CAD build for the part. Positions are in the model's coordinates, mm. Give positions to 0.01 mm unless a question says otherwise; leave off trailing zeros. Write each loop counter-clockwise with the first axis right and the second up, starting at its lowest first coordinate (ties: lowest second). Pieces come first, ordered by that corner, then holes. Notation, with made-up numbers: (-34, 6) - (-23, 6) arc R29 ccw to (-23, 36) - close; hole circle Ø4 at (-18.75, -39). An arc over 180 degrees is marked (long way). Answer as a JSON object with one key per item and string values.
from build123d import *

# Parameters (mm, degrees)
CROQUIS1_R              = 3
SALIENTE_EXTRUIR1_DEPTH = 5
REDONDEO1_R             = 2.99


with BuildPart() as part:
    # Croquis1 → Saliente-Extruir1 (new body)
    with BuildSketch(Plane(origin=(0, 0, 0), x_dir=(1, 0, 0), z_dir=(0, 1, 0))):
        with BuildLine():
            Line((-7.962657019, 208.875039065), (-0.868497325, 213.470388318))
            Line((-0.868497325, 213.470388318), (6.225662369, 208.875039065))
            ThreePointArc((6.225662369, 208.875039065), (10.67506724, 203.378580688), (11.42992133, 196.347332315))
            Line((11.42992133, 196.347332315), (2.131502675, 96.347332315))
            Line((2.131502675, 96.347332315), (-3.868497325, 96.347332315))
            Line((-3.868497325, 96.347332315), (-13.166915979, 196.347332315))
            ThreePointArc((-13.166915979, 196.347332315), (-12.412061889, 203.378580688), (-7.962657019, 208.875039065))
        make_face()
        with Locations(Location((-0.868497325, 198.583153998, 0), (0, 0, 270))):
            Circle(CROQUIS1_R, mode=Mode.SUBTRACT)
    extrude(amount=SALIENTE_EXTRUIR1_DEPTH)

    # Redondeo1
    redondeo1_edges = [part.edges().sort_by_distance(p)[0] for p in [
        (2.131502675, 2.5, -96.347332315),
        (-3.868497325, 2.5, -96.347332315),
    ]]
    fillet(redondeo1_edges, radius=REDONDEO1_R)


solid = part.part
Item 1: Cut at D-D (x = 8.5). Give the cut face in (y, z).
Entries:
{"outline": "(0, -206.86) - (5, -206.86) - (5, -164.84) - (0, -164.84) - close"}
Item 2: Cut at C-C (z = -163.5). Give the cut face in (x, y), and give its area (3 significant figures).
Entries:
{"outline": "(-10.11, 0) - (8.38, 0) - (8.38, 5) - (-10.11, 5) - close", "area": "92.4 mm2"}
Item 3: Cut at B-B (z = -198). Give the cut face in (x, y).
Entries:
{"outline": "(-13.35, 0) - (-3.81, 0) - (-3.81, 5) - (-13.35, 5) - close; (2.07, 0) - (11.62, 0) - (11.62, 5) - (2.07, 5) - close"}
Item 4: Mould opens along Z. For faces 1 (the cylindrical face through (-0.74, 2.46, -201.58)), 2 (the cylindrical face through (-12.45, 2.46, -203.29)), 3 (the flat face through (6.97, 2.46, -148.38)) say: +Z half, -Z half, draft (parallel to the pull), parting line (faces both ways), or undercut.
Entries:
{"face 1": "undercut", "face 2": "parting line", "face 3": "+Z half"}
Item 5: Flat gauge pin, fed straight in: P1, Ø3, axis at y = 4, z = -143.5, coming from the +X side. Where does the tip first touch, or does it go through?
Entries:
{"P1": "x = 6.66"}
Item 6: Cut at A-A (y = 4). Give the cut face in (x, z), and give its area (3 significant figures).
Entries:
{"outline": "(-13.17, -196.35) arc R12.5 ccw to (-7.96, -208.88) - (-0.87, -213.47) - (6.23, -208.88) arc R12.5 ccw to (11.43, -196.35) - (2.38, -99.06) arc R2.99 ccw to (-0.59, -96.35) - (-1.14, -96.35) arc R2.99 ccw to (-4.12, -99.06) - close; hole circle Ø6 at (-0.87, -198.58)", "area": "1,810 mm2"}
Item 7: Probe line 1 (Z direction, x = -1.5, y = 3.2); line 2 (Z direction, x = -1.75, y = 3.3); line 3 (X direction, y = 2.85, z = -135). List the from-to ranges inside material, lowest first. Write a range as from..to.
Entries:
{"line 1": "-213.06..-201.52, -195.65..-96.37", "line 2": "-212.9..-201.45, -195.72..-96.41", "line 3": "-7.46..5.73"}
